Autodesk Inventor part; units mm, degrees
ref_plane "Work Plane1" through (0, 0, 0.2) normal (0, 0, 1) x (1, 0, 0)
ref_plane "YZ Plane" through (0, 0, 0) normal (1, 0, 0) x (0, 1, 0)
ref_plane "XZ Plane" through (0, 0, 0) normal (0, 1, 0) x (-1, 0, 0)
sketch "Sketch1" plane through (0, 0, 0) normal (0, 0, 1) x (1, 0, 0)
  circle A0 centre (0, 0) radius 7.5
  circle A1 centre (0, 0) radius 5
  circle A2 centre (0, 0) radius 5.5
  circle A3 centre (0, 0) radius 7
  dimension "d0" = 15
  dimension "d1" = 10
  dimension "d2" = 0.5
  dimension "d3" = 0.5
extrude "Extrusion1" add sketch "Sketch1" along normal blind 4
ref_plane "Work Plane1" through (0, 0, 0.2) normal (0, 0, 1) x (1, 0, 0)
sketch "Sketch2" plane through (0, 0, 0.2) normal (0, 0, 1) x (1, 0, 0)
  circle A0 centre (0, 0) radius 7
  circle A1 centre (0, 0) radius 7.5
  circle A2 centre (0, 0) radius 5
  circle A3 centre (0, 0) radius 5.5
extrude "Extrusion2" add sketch "Sketch2" along normal blind 3.6 contours A0
properties part number "15x10x4 bearing"
Design review of the part built by this model. Coordinates are the model's own, in mm. A direction names the side the tool comes from. Coordinates: 2 decimals unless noted, no trailing zeros. Order: outer loops, then holes, each group sorted by start corner. A loop starts at its lowest first (then second) coordinate and runs counter-clockwise, first axis right, second up.
1) Clearance check with a flat-ended pin moving along its axis: pin 1 (6 mm diameter, centred on x = 0, y = 0, fed in from -Z). State where the tip first meets the part, or that it passes through.
2) Take a section at B-B, the plane x = 3.5. Give the boundary of the cut face in (y, z).
3) For faces 1 (the flat face through (1.6, -4.9, 0)), 2 (the flat face through (-4, -4, 3.8)), list the 3-axis set-ups (+Z, -Z, +X, -X, +Y, -Y) from which the entire face can be reached by the end or side of a thin tool; tool diameter is ignored.
4) Take a section at A-A, the plane y = 0. Give the boundary of the cut face in (x, z).
5) Wall thickness on line 1 along Y through (x, z) = (0, 3.9); line 2 along Y through (x, z) = (0, 2.05); line 3 along Z through (x, y) = (6.25, 1.75): over which ranges is each line inside the solid? List them lowest first.
6) Take a section at C-C, the plane x = -5.25. Give the boundary of the cut face in (y, z), and give its area (3 significant figures).
7) Mouldability with a two-part tool opening along X and no side actions: class faces 3 (the flat face through (-4, -4, 0.2)), 4 (the cylindrical face through (-1.08, 4.88, 1.97)), 5 (the flat face through (7, 2, 4)), 6 (the cylindrical face through (-7.493, -0.33, 1.972)) as +X half, -X half, draft (parallel to the pull), parting line (faces both ways), or undercut.
8) Take a section at D-D, the plane y = 5.75. Give the boundary of the cut face in (x, z).
Returned:
1. pin 1: passes through
2. outline: (-6.63, 0) - (-6.06, 0) - (-6.06, 0.2) - (-4.24, 0.2) - (-4.24, 0) - (-3.57, 0) - (-3.57, 4) - (-4.24, 4) - (-4.24, 3.8) - (-6.06, 3.8) - (-6.06, 4) - (-6.63, 4) - close; (3.57, 0) - (4.24, 0) - (4.24, 0.2) - (6.06, 0.2) - (6.06, 0) - (6.63, 0) - (6.63, 4) - (6.06, 4) - (6.06, 3.8) - (4.24, 3.8) - (4.24, 4) - (3.57, 4) - close
3. face 1: -Z, +X, -X, +Y, -Y
3. face 2: +Z
4. outline: (-7.5, 0) - (-7, 0) - (-7, 0.2) - (-5.5, 0.2) - (-5.5, 0) - (-5, 0) - (-5, 4) - (-5.5, 4) - (-5.5, 3.8) - (-7, 3.8) - (-7, 4) - (-7.5, 4) - close; (5, 0) - (5.5, 0) - (5.5, 0.2) - (7, 0.2) - (7, 0) - (7.5, 0) - (7.5, 4) - (7, 4) - (7, 3.8) - (5.5, 3.8) - (5.5, 4) - (5, 4) - close
5. line 1: y = -7.5 to -7, -5.5 to -5, 5 to 5.5, 7 to 7.5
5. line 2: y = -7.5 to -5, 5 to 7.5
5. line 3: z = 0.2 to 3.8
6. outline: (-5.36, 0) - (-4.63, 0) - (-4.63, 0.2) - (-1.64, 0.2) - (-1.64, 0) - (1.64, 0) - (1.64, 0.2) - (4.63, 0.2) - (4.63, 0) - (5.36, 0) - (5.36, 4) - (4.63, 4) - (4.63, 3.8) - (1.64, 3.8) - (1.64, 4) - (-1.64, 4) - (-1.64, 3.8) - (-4.63, 3.8) - (-4.63, 4) - (-5.36, 4) - close
6. area: 40.5 mm2
7. face 3: undercut
7. face 4: undercut
7. face 5: draft
7. face 6: parting line
8. outline: (-4.82, 0) - (-3.99, 0) - (-3.99, 0.2) - (3.99, 0.2) - (3.99, 0) - (4.82, 0) - (4.82, 4) - (3.99, 4) - (3.99, 3.8) - (-3.99, 3.8) - (-3.99, 4) - (-4.82, 4) - close
